The listing builds one solid part. Answer for the finished solid, in the listing's coordinates (mm). A direction names the side the tool comes from. Round coordinates to 2 decimals unless told otherwise and drop trailing zeros. Loops run counter-clockwise (first coordinate to the right, second up) from the corner with the lowest first, then second, coordinate; pieces in that order, holes last. Notation, with made-up numbers: (14, 16.25) -> (48, 16.25) arc R19 cw to (48, 29.25) -> close; hole circle Ø11 at (41.25, -21.75). An arc over 180 degrees is marked (long way). Use a Markdown table: item, result. Add a question column.
Q1. For a pull along X with two mould halves and no side action, classify faces 4 (the flat face through (8, 7, 14)), 5 (the cylindrical face through (14.699, 7.591, 0.285)), 6 (the cylindrical face through (14.51, 9.66, 2.7)), 7 (the cylindrical face through (0.285, 0.301, 7.591)) as released by +X, released by -X, zero draft, split by the parting line, or undercut.
Q2. Which of the six approach directions +Z, -Z, +X, -X, +Y, -Y give full straight-line access (tool end or side, diameter ignored) to faces 1 (the cylindrical face through (14.507, 7.108, 5.706)), 2 (the flat face through (11, 11, 14)), 3 (the flat face through (10, 8, 1))?
Q3. Section B-B on z = 6.75 is taken. Give the vertices of the cut face in (x, y).
Q4. Section C-C on y = 6.75 is taken. Give the vertices of the cut face in (x, z), then the cut area to 3 significant figures.
Q5. Consider line 1 (Z direction, x = 5.25, y = 14.75); line 2 (Y direction, x = 6.75, z = 0.5); line 3 (Z direction, x = 9.25, y = 13.5). Determine where each line is inside the solid, lowest interval first.
Q6. Section D-D on y = 13.25 is taken. Give the vertices of the cut face in (x, z).
Q7. Section A-A on y = 4 is taken. Give the vertices of the cut face in (x, z).
Q8. Given pin 1 Ø3 at (x, z) = (4.74, 10.07) entering from +Y; pin 2 Ø1 at (x, y) = (10, 12) entering from -Z, each flat-ended and moving along its own axis, determine where each tip first touches the part or whether it passes through.
from build123d import *

# Parameters (mm, degrees)
F0_W      = 15
F0_H      = 15
F0_R      = 2.6227188779
F1_DEPTH  = 15
F2_R      = 1.4735683416
F2_R_2    = 1.4685130451
F8_DEPTH  = 1
F5_R      = 1.9757699967
F9_DEPTH  = 1
F4_R      = 1.7246799927
F10_DEPTH = 1
F3_R      = 1.7246799927
F11_DEPTH = 1
F7_R      = 1.7246799927
F12_DEPTH = 1
F6_R      = 1.7246799927
F13_DEPTH = 1
F14_R     = 1


with BuildPart() as f1:
    # F0 (on Top) → F1 (new body)
    with BuildSketch(Plane.XY):
        with Locations((7.5, 7.5)):
            Rectangle(F0_W, F0_H)
        with Locations((7.4908491224, 7.7657136135)):
            Circle(F0_R, mode=Mode.SUBTRACT)
        with Locations((7.4908491224, 7.7657136135)):
            Circle(F0_R)
    extrude(amount=F1_DEPTH)

    # F2 (on face) → F8 (cut)
    with BuildSketch(Plane.XZ):
        with Locations((7.3902518488, 4.9254414625)):
            Circle(F2_R)
        with Locations((7.3902518488, 11.0231023282)):
            Circle(F2_R_2)
    extrude(amount=-F8_DEPTH, mode=Mode.SUBTRACT)

    # F5 (on face) → F9 (cut)
    with BuildSketch(Plane(origin=(0, 0, 0), x_dir=(0, -1, 0), z_dir=(-1, 0, 0))):
        with Locations((-7.5194058008, 7.6636224985)):
            Circle(F5_R)
    extrude(amount=-F9_DEPTH, mode=Mode.SUBTRACT)

    # F4 (on face) → F10 (cut)
    with BuildSketch(Plane(origin=(0, 15, 0), x_dir=(-1, 0, 0), z_dir=(0, 1, 0))):
        with Locations((-4.5185647905, 4.4170920737)):
            Circle(F4_R)
        with Locations((-10.6097254902, 10.1456837729)):
            Circle(F4_R)
        with Locations((-10.4646971449, 4.4170920737)):
            Circle(F4_R)
        with Locations((-4.7361063771, 10.0731700659)):
            Circle(F4_R)
    extrude(amount=-F10_DEPTH, mode=Mode.SUBTRACT)

    # F3 (on face) → F11 (cut)
    with BuildSketch(Plane.YZ.offset(15)):
        with Locations((7.4821650051, 7.3897475377)):
            Circle(F3_R)
        with Locations((3.6290215794, 11.4373583347)):
            Circle(F3_R)
        with Locations((11.0254311003, 3.7508946843)):
            Circle(F3_R)
    extrude(amount=-F11_DEPTH, mode=Mode.SUBTRACT)

    # F7 (on face) → F12 (cut)
    with BuildSketch(Plane(origin=(0, 0, 0), x_dir=(1, 0, 0), z_dir=(0, 0, -1))):
        with Locations((5.2725449204, -7.665055804)):
            Circle(F7_R)
        with Locations((5.2115684375, -3.2747397199)):
            Circle(F7_R)
        with Locations((9.9677434191, -12.0858596638)):
            Circle(F7_R)
        with Locations((9.7848139703, -7.7260322869)):
            Circle(F7_R)
        with Locations((9.7848139703, -3.1527867541)):
            Circle(F7_R)
        with Locations((5.2115684375, -11.9943944737)):
            Circle(F7_R)
    extrude(amount=-F12_DEPTH, mode=Mode.SUBTRACT)

    # F6 (on face) → F13 (cut)
    with BuildSketch(Plane.XY.offset(15)):
        with Locations((7.6069538482, 7.2701666504)):
            Circle(F6_R)
        with Locations((11.4286709577, 3.6876818631)):
            Circle(F6_R)
        with Locations((11.2624969333, 11.3061647862)):
            Circle(F6_R)
        with Locations((3.5987806041, 11.1777177081)):
            Circle(F6_R)
        with Locations((3.9099473506, 3.6097485572)):
            Circle(F6_R)
    extrude(amount=-F13_DEPTH, mode=Mode.SUBTRACT)

    # F14
    f14_edges = [f1.edges().sort_by_distance(p)[0] for p in [
        (15, 7.5, 0),
        (7.5, 15, 0),
        (15, 15, 7.5),
        (7.5, 0, 0),
        (0, 7.5, 0),
        (0, 15, 7.5),
        (0, 7.5, 15),
        (0, 0, 7.5),
        (7.5, 0, 15),
        (15, 0, 7.5),
        (15, 7.5, 15),
        (7.5, 15, 15),
    ]]
    fillet(f14_edges, radius=F14_R)


solid = f1.part
Checked values:
| question | item | result |
|---|---|---|
| 1 | face 4 | undercut |
| 1 | face 5 | released by +X |
| 1 | face 6 | zero draft |
| 1 | face 7 | released by -X |
| 2 | face 1 | +X |
| 2 | face 2 | +Z |
| 2 | face 3 | -Z |
| 3 | outline | (0, 1) arc R1 ccw to (1, 0) -> (14, 0) arc R1 ccw to (15, 1) -> (15, 5.88) -> (14, 5.88) -> (14, 9.08) -> (15, 9.08) -> (15, 14) arc R1 ccw to (14, 15) -> (1, 15) arc R1 ccw to (0, 14) -> (0, 9.27) -> (1, 9.27) -> (1, 5.77) -> (0, 5.77) -> close |
| 4 | outline | (0, 1) arc R1 ccw to (1, 0) -> (3.81, 0) -> (3.81, 1) -> (6.73, 1) -> (6.73, 0) -> (8.36, 0) -> (8.36, 1) -> (11.21, 1) -> (11.21, 0) -> (14, 0) arc R1 ccw to (15, 1) -> (15, 5.83) -> (14, 5.83) -> (14, 8.95) -> (15, 8.95) -> (15, 14) arc R1 ccw to (14, 15) -> (9.25, 15) -> (9.25, 14) -> (5.96, 14) -> (5.96, 15) -> (1, 15) arc R1 ccw to (0, 14) -> (0, 9.48) -> (1, 9.48) -> (1, 5.84) -> (0, 5.84) -> close |
| 4 | area | 208 mm2 |
| 5 | line 1 | z = 0.34 to 2.86, 5.98 to 8.43, 11.72 to 14.66 |
| 5 | line 2 | y = 0.13 to 2.5, 4.05 to 6.78, 8.55 to 11.21, 12.77 to 14.87 |
| 5 | line 3 | z = 1 to 15 |
| 6 | outline | (0, 1) arc R1 ccw to (1, 0) -> (4.03, 0) -> (4.03, 1) -> (6.39, 1) -> (6.39, 0) -> (8.7, 0) -> (8.7, 1) -> (11.24, 1) -> (11.24, 0) -> (14, 0) arc R1 ccw to (15, 1) -> (15, 14) arc R1 ccw to (14, 15) -> (1, 15) arc R1 ccw to (0, 14) -> close |
| 7 | outline | (0, 1) arc R1 ccw to (1, 0) -> (3.65, 0) -> (3.65, 1) -> (6.78, 1) -> (6.78, 0) -> (8.28, 0) -> (8.28, 1) -> (11.29, 1) -> (11.29, 0) -> (14, 0) arc R1 ccw to (15, 1) -> (15, 9.75) -> (14, 9.75) -> (14, 13.12) -> (15, 13.12) -> (15, 14) arc R1 ccw to (14, 15) -> (13.12, 15) -> (13.12, 14) -> (9.73, 14) -> (9.73, 15) -> (5.59, 15) -> (5.59, 14) -> (2.23, 14) -> (2.23, 15) -> (1, 15) arc R1 ccw to (0, 14) -> close |
| 8 | pin 1 | stops at y = 14 |
| 8 | pin 2 | stops at z = 1 |
